```python
from build123d import *

# Parameters (mm, degrees)
SKETCH1_W           = 5.6
SKETCH1_H           = 5.4
BOSS_EXTRUDE1_DEPTH = 2
SKETCH3_R           = 0.95
CUT_EXTRUDE2_DEPTH  = 9.5
SKETCH7_R           = 1.2
CUT_EXTRUDE4_DEPTH  = 2.8
SKETCH2_R           = 1.75
BOSS_EXTRUDE2_DEPTH = 20
FILLET2_R           = 1.5
SKETCH8_R           = 0.95
CUT_EXTRUDE5_DEPTH  = 9.5


with BuildPart() as part:
    # Sketch1 → Boss-Extrude1 (new body)
    with BuildSketch(Plane(origin=(0, 0, 0), x_dir=(1, 0, 0), z_dir=(0, 1, 0))):
        Rectangle(SKETCH1_W, SKETCH1_H)
    extrude(amount=BOSS_EXTRUDE1_DEPTH)

    # Sketch3 → Cut-Extrude2 (cut)
    with BuildSketch(Plane.XZ):
        with Locations(Location((0, 0, 0), (0, 0, 270))):
            Circle(SKETCH3_R)
    extrude(amount=-CUT_EXTRUDE2_DEPTH, mode=Mode.SUBTRACT)

    # Sketch7 → Cut-Extrude4 (cut)
    with BuildSketch(Plane.XZ):
        with Locations(Location((0, 0, 0), (0, 0, 270))):
            Circle(SKETCH7_R)
    extrude(amount=-CUT_EXTRUDE4_DEPTH, mode=Mode.SUBTRACT)

    # Sketch2 → Boss-Extrude2 (add)
    with BuildSketch(Plane(origin=(0, 2, 0), x_dir=(1, 0, 0), z_dir=(0, 1, 0))):
        with Locations(Location((0, 0, 0), (0, 0, 90))):
            Circle(SKETCH2_R)
    extrude(amount=BOSS_EXTRUDE2_DEPTH)

    # Fillet2
    fillet2_edges = [part.edges().sort_by_distance(p)[0] for p in [
        (0, 22, 1.75),
    ]]
    fillet(fillet2_edges, radius=FILLET2_R)

    # Sketch8 → Cut-Extrude5 (cut)
    with BuildSketch(Plane.XZ):
        with Locations(Location((0, 0, 0), (0, 0, 270))):
            Circle(SKETCH8_R)
    extrude(amount=-CUT_EXTRUDE5_DEPTH, mode=Mode.SUBTRACT)


solid = part.part
```
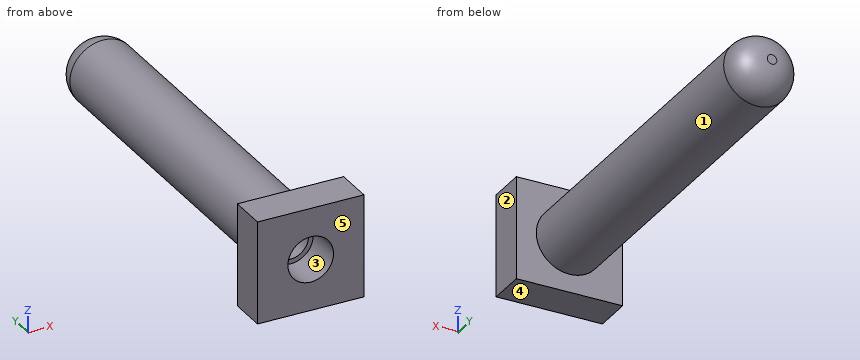
Check sheet for the modelled part. Datum: model origin and axes. Units: mm. Face numbers are marked on the shaded views. A direction names the side the tool comes from. Give positions to 0.01 mm unless a question says otherwise; leave off trailing zeros. Write each loop counter-clockwise with the first axis right and the second up, starting at its lowest first coordinate (ties: lowest second). Pieces come first, ordered by that corner, then holes.
Item 1: Draft check along Z on the marked faces 3, 4 and 5. Enter one of: released by +Z, released by -Z, zero draft, split by the parting line, or undercut.
Item 2: Scan lines: L1, parallel to X at y = 4, z = 0; L2, parallel to X at y = 0.65, z = 0; L3, parallel to Y at x = 2.45, z = -2.1. Record each from-to range of solid material in increasing order.
Item 3: Cross-section at A-A (y = 12.25). Enter the section's corners in (x, z), and give its area (3 significant figures).
Item 4: Cross-section at B-B (x = -2.25). Enter the section's corners in (y, z), and give its area (3 significant figures).
Item 5: Access from +Z, -Z, +X, -X, +Y, -Y to the whole of each face (thin tool, end or side, straight path). Record for the marked faces 1 and 2.
Item 6: Gauge pin test, flat ends, axial feed: pin 1 (3 mm diameter, centred on y = 19, z = -1.5, fed in from +X); pin 2 (3 mm diameter, centred on y = 10.5, z = 0, fed in from -X); pin 3 (1.4 mm diameter, centred on x = 0, z = 0, fed in from -Y). Record the tip position at first contact, or that the pin passes through.
Report:
1. face 3: undercut
1. face 4: released by -Z
1. face 5: zero draft
2. L1: x = -1.75 to -0.95, 0.95 to 1.75
2. L2: x = -2.8 to -1.2, 1.2 to 2.8
2. L3: y = 0 to 2
3. outline: circle Ø3.5 at (0, 0)
3. area: 9.62 mm2
4. outline: (0, -2.7) - (2, -2.7) - (2, 2.7) - (0, 2.7) - close
4. area: 10.8 mm2
5. face 1: +Y
5. face 2: +Z, -Z, +X, +Y, -Y
6. pin 1: stops at x = 1.75
6. pin 2: stops at x = -1.75
6. pin 3: stops at y = 9.5
